Geometry check sheet. Reference: drawing and pictorial views, mm from the part's lowest x, y, z. A direction names the side the tool comes from. Round coordinates to 2 decimals unless told otherwise and drop trailing zeros. Loops run counter-clockwise (first coordinate to the right, second up) from the corner with the lowest first, then second, coordinate; pieces in that order, holes last. Notation, with made-up numbers: (-1.75, 58) -> (30.25, 58) arc R27 ccw to (30.25, 90) -> close; hole circle Ø6 at (3.5, 41.25). An arc over 180 degrees is marked (long way). Use one line per item in the form item = value. Start each with the question number.
(1) Sectioned sample at C-C (y = 14.5). Record the cut outline in (x, z).
(2) Go/stop test with flat-tipped pins: pin 1 (9.5 mm diameter, centred on x = 23.5, z = 17.5, fed in from -Y); pin 2 (1 mm diameter, centred on x = 33.5, y = 7.5, fed in from +Z); pin 3 (10 mm diameter, centred on x = 17.5, y = 5.5, fed in from +Z); pin 4 (8 mm diameter, centred on y = 12, z = 19.5, fed in from +X). Record where each tip stops, or that it passes through.
(3) Sectioned sample at B-B (x = 14). Record the cut outline in (y, z).
(4) Sectioned sample at D-D (x = 28). Record the cut outline in (y, z).
(5) Set-up check for the marked faces 1 and 2: record each of +Z, -Z, +X, -X, +Y, -Y from which the full face is reachable in a straight line by a thin tool's end or side.
(6) Material ranges on probe 1 along Y at (x, z) = (21, 17); probe 2 along Z at (x, y) = (15.5, 6.75); probe 3 along X at (y, z) = (8.5, 12), recorded low to high. Write a range as [from, to].
(7) Sectioned sample at A-A (z = 4). Record the cut outline in (x, y), and give its area (3 significant figures).
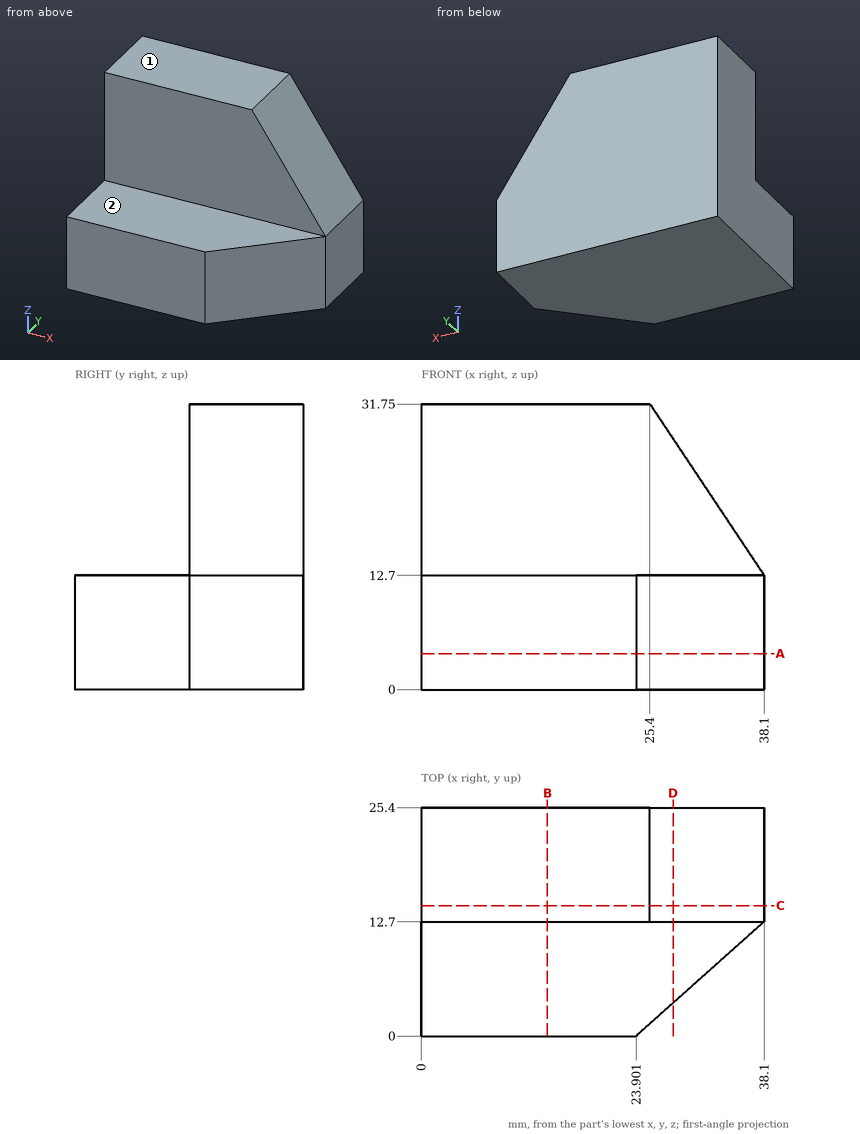
Checks:
q1.outline = (0, 0) -> (38.1, 0) -> (38.1, 12.7) -> (25.4, 31.75) -> (0, 31.75) -> close
q2.pin_1 = 12.7
q2.pin_2 = through
q2.pin_3 = 12.7
q2.pin_4 = 36.19
q3.outline = (0, 0) -> (25.4, 0) -> (25.4, 31.75) -> (12.7, 31.75) -> (12.7, 12.7) -> (0, 12.7) -> close
q4.outline = (3.67, 0) -> (25.4, 0) -> (25.4, 27.85) -> (12.7, 27.85) -> (12.7, 12.7) -> (3.67, 12.7) -> close
q5.face_1 = +Z, +X, -X, +Y, -Y
q5.face_2 = +Z, +X, -X, -Y
q6.probe_1 = [12.7, 25.4]
q6.probe_2 = [0, 12.7]
q6.probe_3 = [0, 33.4]
q7.outline = (0, 0) -> (23.9, 0) -> (38.1, 12.7) -> (38.1, 25.4) -> (0, 25.4) -> close
q7.area = 878 mm2
